```python
from build123d import *

# Parameters (mm, degrees)
SKETCH_1_R          = 18.5
EXTRUDE_1_DEPTH     = 4
SKETCH_2_R          = 5
SKETCH_2_R_2        = 1.5
CUT_EXTRUDE_1_DEPTH = 10
SKETCH_4_R          = 2
CUT_EXTRUDE_2_DEPTH = 4
SKETCH_5_W          = 25
SKETCH_5_H          = 5
EXTRUDE_2_DEPTH     = 4
SKETCH_6_R          = 1
CUT_EXTRUDE_3_DEPTH = 10
FILLET_2_R          = 1
CUT_EXTRUDE_START   = -5
CUT_EXTRUDE_4_DEPTH = 5
EXTRUDE_1_2_DEPTH   = 4
FILLET_3_R          = 2
FILLET_4_R          = 3
FILLET_5_R          = 1
SKETCH_10_R         = 3
SKETCH_10_R_2       = 1.5
EXTRUDE_3_DEPTH     = 4
FILLET_6_R          = 3
CUT_EXTRUDE_5_DEPTH = 4
FILLET_7_R          = 5


with BuildPart() as part:
    # 草图1 → Extrude 1 (new body)
    with BuildSketch(Plane(origin=(0, 0, 0), x_dir=(1, 0, 0), z_dir=(0, 1, 0))):
        with BuildLine():
            ThreePointArc((-23.869289328, -2.501404997), (0, -24), (23.869289328, -2.501404997))
            Line((23.869289328, -2.501404997), (31.047959561, 66))
            Line((31.047959561, 66), (-31.047959561, 66))
            Line((-31.047959561, 66), (-23.869289328, -2.501404997))
        make_face()
        with Locations(Location((0, 0, 0), (0, 0, 270))):
            Circle(SKETCH_1_R, mode=Mode.SUBTRACT)
    extrude(amount=EXTRUDE_1_DEPTH)

    # 草图2 → 切除-拉伸1 (cut)
    with BuildSketch(Plane(origin=(0, 4, 0), x_dir=(1, 0, 0), z_dir=(0, 1, 0))):
        with Locations((0, -31.5)):
            Circle(SKETCH_2_R)
        with Locations(Location((0, 23, 0), (0, 0, 270))):
            Circle(SKETCH_2_R_2)
        with Locations((19.918584287, -11.5)):
            Circle(SKETCH_2_R_2)
        with Locations((-19.918584287, -11.5)):
            Circle(SKETCH_2_R_2)
    extrude(amount=-CUT_EXTRUDE_1_DEPTH, mode=Mode.SUBTRACT)

    # 草图4 → 切除-拉伸2 (cut)
    with BuildSketch(Plane(origin=(0, 4, 0), x_dir=(1, 0, 0), z_dir=(0, 1, 0))):
        with Locations(Location((-25, 61, 0), (0, 0, 270))):
            Circle(SKETCH_4_R)
        with Locations(Location((0, 61, 0), (0, 0, 270))):
            Circle(SKETCH_4_R)
        with Locations(Location((25, 61, 0), (0, 0, 270))):
            Circle(SKETCH_4_R)
    extrude(amount=-CUT_EXTRUDE_2_DEPTH, mode=Mode.SUBTRACT)

    # 草图5 → 凸台-拉伸2 (add)
    with BuildSketch(Plane(origin=(0, 4, 0), x_dir=(1, 0, 0), z_dir=(0, 1, 0))):
        with Locations((0, 68.5)):
            Rectangle(SKETCH_5_W, SKETCH_5_H)
    extrude(amount=-EXTRUDE_2_DEPTH)

    # 草图6 → 切除-拉伸3 (cut)
    with BuildSketch(Plane(origin=(0, 4, 0), x_dir=(1, 0, 0), z_dir=(0, 1, 0))):
        with Locations((-13.5, 66)):
            Circle(SKETCH_6_R)
        with Locations((13.5, 66)):
            Circle(SKETCH_6_R)
    extrude(amount=-CUT_EXTRUDE_3_DEPTH, mode=Mode.SUBTRACT)

    # 圆角2
    fillet_2_edges = [part.edges().sort_by_distance(p)[0] for p in [
        (12.5, 2, -71),
        (-12.5, 2, -71),
    ]]
    fillet(fillet_2_edges, radius=FILLET_2_R)

    # 草图7 → 切除-拉伸4 (cut)
    with BuildSketch(Plane(origin=(0, 4, 0), x_dir=(1, 0, 0), z_dir=(0, 1, 0)).offset(CUT_EXTRUDE_START)):
        with BuildLine():
            Line((-19.556490884, 13.911997136), (-23.967143386, 56))
            Line((-23.967143386, 56), (23.967143386, 56))
            Line((23.967143386, 56), (19.556490884, 13.911997136))
            ThreePointArc((19.556490884, 13.911997136), (12.266476425, 20.628464705), (2.884021557, 23.826086957))
            ThreePointArc((2.884021557, 23.826086957), (0, 26), (-2.884021557, 23.826086957))
            ThreePointArc((-2.884021557, 23.826086957), (-12.266476425, 20.628464705), (-19.556490884, 13.911997136))
        make_face()
    extrude(amount=CUT_EXTRUDE_4_DEPTH, mode=Mode.SUBTRACT)

    # 草图8 → Extrude 1 2 (add)
    with BuildSketch(Plane(origin=(0, 4, 0), x_dir=(1, 0, 0), z_dir=(0, 1, 0))):
        Polygon((-26.265493929, 55.016341125), (-9.577426219, 16.024135141), (-4.980725133, 17.991452891), (-21.668792843, 56.983658875), align=None)
        Polygon((21.668792843, 56.983658875), (4.980725133, 17.991452891), (9.577426219, 16.024135141), (26.265493929, 55.016341125), align=None)
    extrude(amount=-EXTRUDE_1_2_DEPTH)

    # 圆角3
    fillet_3_edges = [part.edges().sort_by_distance(p)[0] for p in [
        (-11.690103776, 2, -20.960474081),
        (-7.09340269, 2, -22.927791832),
        (11.690103776, 2, -20.960474081),
        (7.09340269, 2, -22.927791832),
    ]]
    fillet(fillet_3_edges, radius=FILLET_3_R)

    # 圆角4
    fillet_4_edges = [part.edges().sort_by_distance(p)[0] for p in [
        (-2.884021557, 2, -23.826086957),
        (2.884021557, 2, -23.826086957),
    ]]
    fillet(fillet_4_edges, radius=FILLET_4_R)

    # 圆角5
    fillet_5_edges = [part.edges().sort_by_distance(p)[0] for p in [
        (-19.556490884, 2, -13.911997136),
        (19.556490884, 2, -13.911997136),
        (-21.247801891, 2, -56),
        (-23.085380037, 2, -47.585902918),
        (21.247801891, 2, -56),
        (23.085380037, 2, -47.585902918),
    ]]
    fillet(fillet_5_edges, radius=FILLET_5_R)

    # 草图10 → 凸台-拉伸3 (add)
    # profile 1 of 2: a face of its own
    with BuildSketch(Plane(origin=(0, 4, 0), x_dir=(1, 0, 0), z_dir=(0, 1, 0))):
        with Locations((-19.918584287, -11.5)):
            Circle(SKETCH_10_R)
        with Locations(Location((-19.918584287, -11.5, 0), (0, 0, 270))):
            Circle(SKETCH_10_R_2, mode=Mode.SUBTRACT)
    # profile 2 of 2: a face of its own
    with BuildSketch(Plane(origin=(0, 4, 0), x_dir=(1, 0, 0), z_dir=(0, 1, 0))):
        with Locations((19.918584287, -11.5)):
            Circle(SKETCH_10_R)
        with Locations(Location((19.918584287, -11.5, 0), (0, 0, 270))):
            Circle(SKETCH_10_R_2, mode=Mode.SUBTRACT)
    extrude(amount=-EXTRUDE_3_DEPTH)

    # 圆角6
    fillet_6_edges = [part.edges().sort_by_distance(p)[0] for p in [
        (-22.076007356, 2, 9.415407545),
        (-19.191985799, 2, 14.410679412),
        (22.076007356, 2, 9.415407545),
        (19.191985799, 2, 14.410679412),
    ]]
    fillet(fillet_6_edges, radius=FILLET_6_R)

    # 草图11 → 切除-拉伸5 (cut)
    with BuildSketch(Plane(origin=(0, 4, 0), x_dir=(1, 0, 0), z_dir=(0, 1, 0))):
        Polygon((-30, 66), (-30, 56), (-31.047959561, 66), align=None)
        Polygon((30, 66), (31.047959561, 66), (30, 56), align=None)
    extrude(amount=-CUT_EXTRUDE_5_DEPTH, mode=Mode.SUBTRACT)

    # 圆角7
    fillet_7_edges = [part.edges().sort_by_distance(p)[0] for p in [
        (-30, 2, -56),
        (30, 2, -56),
    ]]
    fillet(fillet_7_edges, radius=FILLET_7_R)


solid = part.part
```
The listing builds one solid part. Answer for the finished solid, in the listing's coordinates (mm). A direction names the side the tool comes from. Coordinates: 2 decimals unless noted, no trailing zeros. Loops run counter-clockwise (first coordinate to the right, second up) from the corner with the lowest first, then second, coordinate; pieces in that order, holes last. Notation, with made-up numbers: (61.5, 27.25) - (105.5, 27.25) arc R14 cw to (105.5, 52.25) - close; hole circle Ø4 at (5, -11.75). An arc over 180 degrees is marked (long way). Use a Markdown table: item, result. Add a question column.
1) Find the intervals of material crossed by line 1 (X direction, y = 2.3, z = -61); line 2 (Z direction, x = 4, y = 2.8); line 3 (Z direction, x = 8, y = 1.25), in increasing order.
2) The part is cut by section B-B, the plane z = 5. Give the vertices of the cut face in (x, y), and give its area (3 significant figures).
3) The part is cut by section A-A, the plane z = -61. Give the vertices of the cut face in (x, y).
4) For faces 1 (the flat face through (-14.124, 2.028, -39.356)), 2 (the flat face through (-30, 2, -61)), 3 (the flat face through (22, 2, -66)), 4 (the cylindrical face through (23.39, 1.97, 5.37)), 5 (the flat face through (-22, 2, -66)), determine the directions among +Z, -Z, +X, -X, +Y, -Y from which every point of the face is accessible in a straight line to the end or side of a thin tool.
5) The mould has two halves that part along X. Classify faces 6 (the flat face through (30, 2, -61)), 7 (the flat face through (0, 2, -71)), 8 (the cylindrical face through (0.07, 2.03, -24.5)), 9 (the cylindrical face through (0, 2, -26)): released by +X, released by -X, zero draft, split by the parting line, or undercut.
6) The part is cut by section D-D, the plane y = 2.25. State how many separate pieces and enclosed holes the cut face has, and give its area (3 significant figures).
7) The part is cut by section C-C, the plane x = 25. Give the vertices of the cut face in (y, z), and give its area (3 significant figures).
8) Given pin 1 (2 mm diameter, centred on y = 2.5, z = -68, fed in from -X), flat-ended and moving along its own axis, determine where the tip first touches the part or whether it passes through.
Here are the results:
| question | item | result |
|---|---|---|
| 1 | line 1 | x = -30 to -27, -23 to -2, 2 to 23, 27 to 30 |
| 1 | line 2 | z = -71 to -56, -23.68 to -18.06, 18.06 to 23.66 |
| 1 | line 3 | z = -71 to -56, -25.05 to -16.68, 16.68 to 22.63 |
| 2 | outline | (-23.47, 0) - (-17.81, 0) - (-17.81, 4) - (-23.47, 4) - close; (17.81, 0) - (23.47, 0) - (23.47, 4) - (17.81, 4) - close |
| 2 | area | 45.3 mm^2 |
| 3 | outline | (-30, 0) - (-27, 0) - (-27, 4) - (-30, 4) - close; (-23, 0) - (-2, 0) - (-2, 4) - (-23, 4) - close; (2, 0) - (23, 0) - (23, 4) - (2, 4) - close; (27, 0) - (30, 0) - (30, 4) - (27, 4) - close |
| 4 | face 1 | +Y, -Y |
| 4 | face 2 | +Z, -Z, -X, +Y, -Y |
| 4 | face 3 | -Z, +X, +Y, -Y |
| 4 | face 4 | +X, +Y, -Y |
| 4 | face 5 | -Z, -X, +Y, -Y |
| 5 | face 6 | released by +X |
| 5 | face 7 | zero draft |
| 5 | face 8 | undercut |
| 5 | face 9 | undercut |
| 6 | separate pieces | 1 |
| 6 | enclosed holes | 10 |
| 6 | area | 2,360 mm^2 |
| 7 | outline | (0, -66) - (4, -66) - (4, -63) - (0, -63) - close; (0, -59) - (4, -59) - (4, -8.29) - (0, -8.29) - close |
| 7 | area | 215 mm^2 |
| 8 | pin 1 | stops at x = -12.5 |
